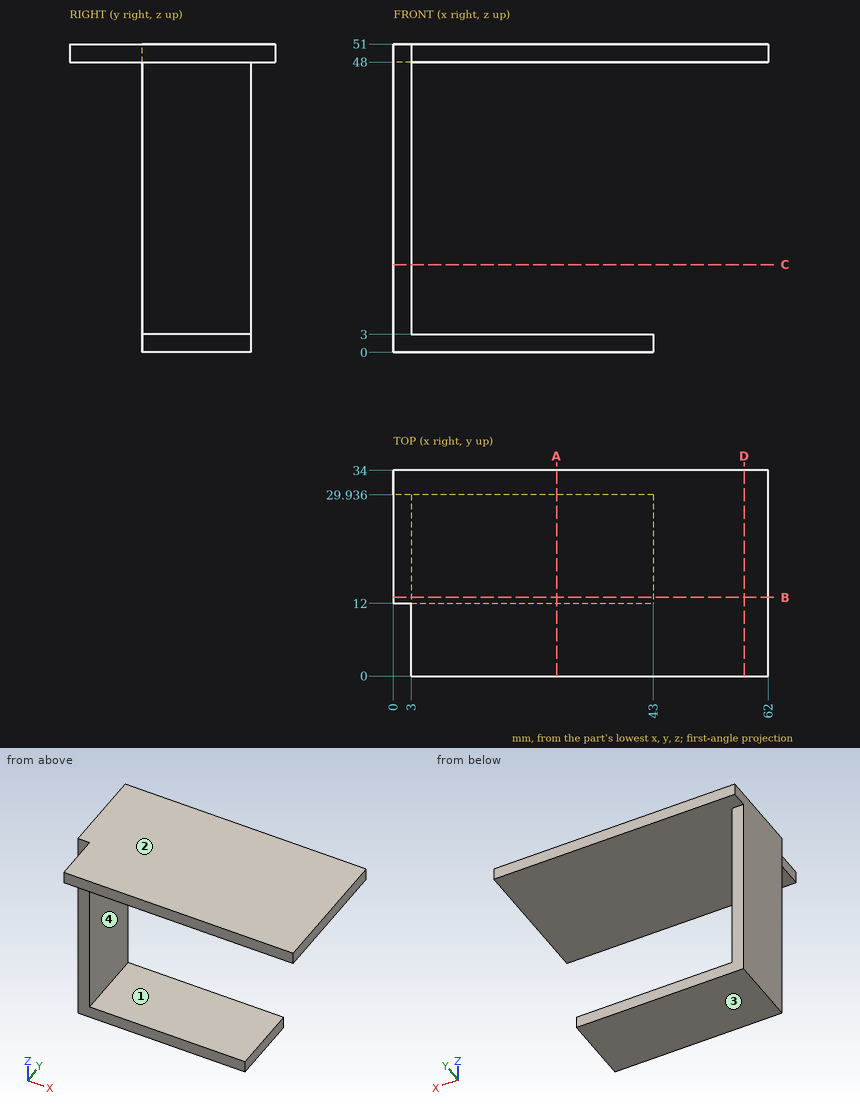
Answer from the drawing. Dimensions are ordinates in mm from the lowest x, y and z of the part. Give positions to 0.01 mm unless a question says otherwise; leave off trailing zeros. Order: outer loops, then holes, each group sorted by start corner. A loop starts at its lowest first (then second) coordinate and runs counter-clockwise, first axis right, second up. Notation, with made-up numbers: (87, 25.25) -> (135, 25.25) arc R18 cw to (135, 45.25) -> close; hole circle Ø9 at (-36.5, 17.5). An arc over 180 degrees is marked (long way). Answer as a JSON object with one key per item and string values. Group by question number.
1. Section D-D on x = 58 is taken. Determine the outline of the cut face in (y, z), plus the area to 3 significant figures.
2. Flat-ended cylindrical pins translate along their axes: pin 1 Ø2.5 at (y, z) = (6, 50) entering from -X; pin 2 Ø3 at (x, y) = (12, 16) entering from -Z; pin 3 Ø3.5 at (y, z) = (20, 2) entering from +X; pin 4 Ø4 at (y, z) = (22, 27.5) entering from +X. Find the tip coordinate at first contact, or state that the pin passes through.
3. Consider line 1 along Z through (x, y) = (9.5, 29); line 2 along X through (y, z) = (23.5, 19); line 3 along Z through (x, y) = (55, 12). Determine where each line is inside the solid, lowest interval first. Write a range as [from, to].
4. Section C-C on z = 14.5 is taken. Determine the outline of the cut face in (x, y) (1 decimal).
5. Section A-A on x = 27 is taken. Determine the outline of the cut face in (y, z) (1 decimal), plus the area to 3 significant figures.
6. The mould has two halves that part along Z. Classify the marked faces 1, 2, 3 and 4: released by +Z, released by -Z, zero draft, split by the parting line, or undercut.
7. Section B-B on y = 13 is taken. Determine the outline of the cut face in (x, z).
Result sheet:
{
 "1": {"outline": "(0, 48) -> (34, 48) -> (34, 51) -> (0, 51) -> close", "area": "102 mm^2"},
 "2": {"pin 1": "stops at x = 3", "pin 2": "stops at z = 0", "pin 3": "stops at x = 43", "pin 4": "stops at x = 3"},
 "3": {"line 1": "z = [0, 3], [48, 51]", "line 2": "x = [0, 3]", "line 3": "z = [48, 51]"},
 "4": {"outline": "(0, 12) -> (3, 12) -> (3, 29.9) -> (0, 29.9) -> close"},
 "5": {"outline": "(0, 48) -> (34, 48) -> (34, 51) -> (0, 51) -> close; (12, 0) -> (29.9, 0) -> (29.9, 3) -> (12, 3) -> close", "area": "156 mm^2"},
 "6": {"face 1": "undercut", "face 2": "released by +Z", "face 3": "released by -Z", "face 4": "undercut"},
 "7": {"outline": "(0, 0) -> (43, 0) -> (43, 3) -> (3, 3) -> (3, 48) -> (62, 48) -> (62, 51) -> (0, 51) -> close"}
}
